Work out the finished part from the listing and answer in its coordinate system (mm). Face numbers are marked on the shaded views. A direction names the side the tool comes from. Coordinates: 2 decimals unless noted, no trailing zeros. Write each loop counter-clockwise with the first axis right and the second up, starting at its lowest first coordinate (ties: lowest second). Pieces come first, ordered by that corner, then holes. Notation, with made-up numbers: M -13.5,-25.5 L 12.5,-25.5 A15 ccw 12.5,3.5 Z; hole C 36,84 d8. An arc over 180 degrees is marked long. Use CSV: the item, a comma, the result in double quotes.
from build123d import *

# Parameters (mm, degrees)
F2_SIZE2 = 1
F2_SIZE  = 1
F3_R     = 3
F4_DEPTH = 12.5


with BuildPart() as f1:
    # F0 (on Front) → F1 (revolve)
    with BuildSketch(Plane.XZ):
        Polygon((-4, 65), (-4, 3), (-3, 3), (-3, 0), (0, 0), (0, 80), (-6, 80), (-6, 65), align=None)
    revolve(axis=Axis((0, 0, 40), (0, 0, -1)))

    # F2
    f2_edges = [f1.edges().sort_by_distance(p)[0] for p in [
        (6, 0, 80),
        (6, 0, 65),
    ]]
    chamfer(f2_edges, length=F2_SIZE, length2=F2_SIZE2)

    # F3 (on Right) → F4 (cut, symmetric)
    with BuildSketch(Plane.YZ):
        with Locations((0, 72.5)):
            Circle(F3_R)
    extrude(amount=F4_DEPTH, both=True, mode=Mode.SUBTRACT)


solid = f1.part
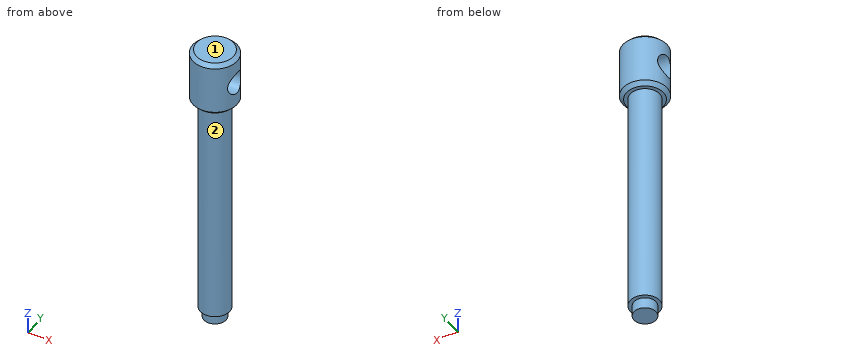
Item 1: The part is cut by section B-B (x = 0). Write down the section's boundary in (y, z).
Answer:
outline,"M -6,66 L -5,65 L -4,65 L -4,3 L -3,3 L -3,0 L 3,0 L 3,3 L 4,3 L 4,65 L 5,65 L 6,66 L 6,79 L 5,80 L -5,80 L -6,79 Z; hole C 0,72.5 d6"
Item 2: A tool of negligible diameter and unlimited length cuts with its end or side. For the marked faces 1 and 2, from which of +Z, -Z, +X, -X, +Y, -Y can it reach the whole face along a straight path? Write none if from no direction.
Answer:
face 1,"+Z, +X, -X, +Y, -Y"
face 2,"-Z"
Item 3: The part is cut by section C-C (z = 37.5). Write down the section's boundary in (x, y).
Answer:
outline,"C 0,0 d8"
Item 4: The part is cut by section A-A (y = 0). Write down the section's boundary in (x, z), then the cut area to 3 significant figures.
Answer:
outline,"M -6,66 L -5,65 L -4,65 L -4,3 L -3,3 L -3,0 L 3,0 L 3,3 L 4,3 L 4,65 L 5,65 L 6,66 L 6,69.5 L -6,69.5 Z; M -6,75.5 L 6,75.5 L 6,79 L 5,80 L -5,80 L -6,79 Z"
area,"620 mm2"
Item 5: The part is cut by section D-D (z = 72.5). Write down the section's boundary in (x, y), then the cut area to 3 significant figures.
Answer:
outline,"M -5.2,-3 A6 ccw 5.2,-3 Z; M -5.2,3 L 5.2,3 A6 ccw Z"
area,"44.2 mm2"
Item 6: Given pin 1 (2 mm diameter, centred on x = 3.5, y = 2, fed in from -Z); pin 2 (2 mm diameter, centred on y = 1.5, z = 42.5, fed in from -X); pin 3 (1 mm diameter, centred on y = 4, z = 34, fed in from +X), each flat-ended and moving along its own axis, determine where each tip first touches the part or whether it passes through.
Answer:
pin 1,"stops at z = 3"
pin 2,"stops at x = -3.97"
pin 3,"stops at x = 1.94"
Item 7: Consider probe 1 along Z at (x, y) = (-0.75, 0); probe 2 along Z at (x, y) = (5.75, 1); probe 3 along Y at (x, z) = (4, 74.5). Determine where each line is inside the solid, lowest interval first.
Answer:
probe 1,"z = 0 to 69.5, 75.5 to 80"
probe 2,"z = 65.84 to 69.67, 75.33 to 79.16"
probe 3,"y = -4.47 to -2.24, 2.24 to 4.47"
